```python
from build123d import *

# Parameters (mm, degrees)
SKETCH_1_W      = 8
SKETCH_1_H      = 3
EXTRUDE_1_DEPTH = 3


with BuildPart() as part:
    # 草图1 → 凸台-拉伸1 (new body)
    with BuildSketch(Plane(origin=(0, 0, 0), x_dir=(1, 0, 0), z_dir=(0, 1, 0))):
        Polygon((-17.5, 21.5), (-25.5, 21.5), (-25.5, 7.5), (-22.5, 7.5), (-22.5, -7.5), (-25.5, -7.5), (-25.5, -21.5), (-17.5, -21.5), (-9.5, -21.5), (9.5, -21.5), (17.5, -21.5), (25.5, -21.5), (25.5, -7.5), (22.5, -7.5), (22.5, 7.5), (25.5, 7.5), (25.5, 21.5), (17.5, 21.5), (9.5, 21.5), (-9.5, 21.5), align=None)
        with Locations((-13.5, 23)):
            Rectangle(SKETCH_1_W, SKETCH_1_H)
        with Locations((13.5, 23)):
            Rectangle(SKETCH_1_W, SKETCH_1_H)
        with Locations((13.5, -23)):
            Rectangle(SKETCH_1_W, SKETCH_1_H)
        with Locations((-13.5, -23)):
            Rectangle(SKETCH_1_W, SKETCH_1_H)
    extrude(amount=EXTRUDE_1_DEPTH)


solid = part.part
```
Geometry: final body of the model. Coordinates: model frame, mm. A direction names the side the tool comes from. Round coordinates to 2 decimals unless told otherwise and drop trailing zeros. Write each loop counter-clockwise with the first axis right and the second up, starting at its lowest first coordinate (ties: lowest second). Pieces come first, ordered by that corner, then holes.
Item 1: Section query C-C (x = -20). Return loops of the section in (y, z), plus the area to 3 significant figures.
Item 2: Section query A-A (y = 0.85). Return loops of the section in (x, z).
Item 3: Pin query (flat end, axial travel): P1, Ø0.9, axis at y = 1, z = -0.5, coming from the -X side; P2, Ø0.9, axis at x = -22.5, y = 1.5, coming from the -Z side; P3, Ø1.5, axis at y = 1, z = -23.5, coming from the +X side. Return the tip coordinate at first contact, or that it passes through.
Item 4: Set-up query: faces 4 (the face through (9.5, 1, -23)), 5 (the face through (-22.5, 1, 0)), 6 (the face through (-22, 1, 21.5)), 7 (the face through (-17.5, 1, -23)), 8 (the face through (0, 1, 21.5)). Return all of +Z, -Z, +X, -X, +Y, -Y with unobstructed straight access to the full face (end or side cutting, diameter ignored); none if empty.
Item 5: Mould query, pull axis Z, two halves, no side actions, for faces 1 (the face through (-24, 1, -7.5)), 2 (the face through (-14, 1, -24.5)), 3 (the face through (-17.5, 1, 23)). Classes: +Z half, -Z half, draft (parallel to the pull), parting line (faces both ways), or undercut.
Item 6: Material intervals for L1, parallel to X at y = 0.5, z = 22; L2, parallel to Z at x = 23.5, y = 1.8; L3, parallel to X at y = 2.4, z = -7, sorted ascending.
Item 7: Section query B-B (z = 3). Return loops of the section in (x, y).
Completed:
1. outline: (0, -21.5) - (3, -21.5) - (3, 21.5) - (0, 21.5) - close
1. area: 129 mm2
2. outline: (-25.5, -21.5) - (-17.5, -21.5) - (-17.5, -24.5) - (-9.5, -24.5) - (-9.5, -21.5) - (9.5, -21.5) - (9.5, -24.5) - (17.5, -24.5) - (17.5, -21.5) - (25.5, -21.5) - (25.5, -7.5) - (22.5, -7.5) - (22.5, 7.5) - (25.5, 7.5) - (25.5, 21.5) - (17.5, 21.5) - (17.5, 24.5) - (9.5, 24.5) - (9.5, 21.5) - (-9.5, 21.5) - (-9.5, 24.5) - (-17.5, 24.5) - (-17.5, 21.5) - (-25.5, 21.5) - (-25.5, 7.5) - (-22.5, 7.5) - (-22.5, -7.5) - (-25.5, -7.5) - close
3. P1: stops at x = -22.5
3. P2: stops at z = -21.5
3. P3: stops at x = 17.5
4. face 4: -Z, +Y, -Y
4. face 5: -X, +Y, -Y
4. face 6: +Z, -X, +Y, -Y
4. face 7: -Z, -X, +Y, -Y
4. face 8: +Z, +Y, -Y
5. face 1: undercut
5. face 2: -Z half
5. face 3: draft
6. L1: x = -17.5 to -9.5, 9.5 to 17.5
6. L2: z = -21.5 to -7.5, 7.5 to 21.5
6. L3: x = -22.5 to 22.5
7. outline: (-22.5, 0) - (22.5, 0) - (22.5, 3) - (-22.5, 3) - close
